```python
from build123d import *

# Parameters (mm, degrees)
SKETCH1_R               = 12.5
SKETCH1_R_2             = 6
BOSS_EXTRUDE1_DEPTH     = 18
SKETCH2_W               = 15
SKETCH2_H               = 15
BOSS_EXTRUDE2_DEPTH     = 25
BOSS_EXTRUDE3_DEPTH     = 20
CHAMFER1_SIZE           = 3
SKETCH4_R               = 5
BOSS_EXTRUDE4_DEPTH     = 15
CUT_EXTRUDE2_DEPTH      = 64.876834612
CUT_EXTRUDE2_DEPTH_BACK = 64.876834612
SKETCH1_3_R             = 6


with BuildPart() as part:
    # Sketch1 → Boss-Extrude1 (new body)
    with BuildSketch(Plane(origin=(0, 0, 0), x_dir=(0, 0, -1), z_dir=(1, 0, 0))):
        Circle(SKETCH1_R)
        Circle(SKETCH1_R_2, mode=Mode.SUBTRACT)
    extrude(amount=BOSS_EXTRUDE1_DEPTH)

    # Sketch2 → Boss-Extrude2 (add)
    with BuildSketch(Plane.XY):
        with Locations((9.060136008, 0)):
            Rectangle(SKETCH2_W, SKETCH2_H)
    extrude(amount=BOSS_EXTRUDE2_DEPTH)

    # Sketch3 → Boss-Extrude3 (add)
    with BuildSketch(Plane.XY.offset(25)):
        Polygon((12.266098975, 5.700421756), (5.666853814, 5.671037358), (2.392678869, -0.058768796), (5.717749085, -5.759190552), (12.316994245, -5.729806154), (15.591169191, 0), align=None)
    extrude(amount=BOSS_EXTRUDE3_DEPTH)

    # Chamfer1
    chamfer1_edges = [part.edges().sort_by_distance(p)[0] for p in [
        (1.560136008, -7.5, 17.5),
        (16.560136008, 7.5, 17.5),
        (1.560136008, 7.5, 17.5),
        (16.560136008, -7.5, 17.5),
    ]]
    chamfer(chamfer1_edges, length=CHAMFER1_SIZE)

    # Sketch4 → Boss-Extrude4 (add)
    with BuildSketch(Plane.XY.offset(45)):
        with Locations((9.066652134, 0)):
            Circle(SKETCH4_R)
    extrude(amount=BOSS_EXTRUDE4_DEPTH)

    # Sketch1<3> → Cut-Extrude2 (cut, two sides: drawn at the far end of the back side and taken through both)
    with BuildSketch(Plane(origin=(0, 0, 0), x_dir=(0, 0, -1), z_dir=(1, 0, 0)).offset(-CUT_EXTRUDE2_DEPTH_BACK)):
        Circle(SKETCH1_3_R)
    extrude(amount=CUT_EXTRUDE2_DEPTH + CUT_EXTRUDE2_DEPTH_BACK, mode=Mode.SUBTRACT)


solid = part.part
```
Here's how the part is built. I have some questions about the finished solid (model axes, mm). A direction names the side the tool comes from. Give positions to 0.01 mm unless a question says otherwise; leave off trailing zeros. Order: outer loops, then holes, each group sorted by start corner. A loop starts at its lowest first (then second) coordinate and runs counter-clockwise, first axis right, second up. Notation, with made-up numbers: (39.5, 66) - (89.5, 66) arc R26 cw to (89.5, 82) - close; hole circle Ø3 at (47, -18.5). An arc over 180 degrees is marked (long way). Answer as a JSON object with one key per item and string values. Group by question number.
Item 1: If we section it at C-C on z = 19.5: Please give me the cut outline in (x, y), and give its area (3 significant figures).
Item 2: If we mould it in two halves opening along Z, with no side actions, what happens to faces 1 (the cylindrical face through (9, 0, 6)), 2 (the flat face through (1.56, 0, 18)), 3 (the flat face through (7, -5, 45))? For each: pulls with the +Z half, pulls with the -Z half, needs draft (parallel to the pull), parting line crosses it, or undercut.
Item 3: For P1, Ø8, axis at y = -1, z = 28, coming from the +X side; P2, Ø3, axis at y = -8.5, z = 37.5, coming from the -X side; P3, Ø7, axis at y = -0.5, z = 17.5, coming from the -X side; P4, Ø4.5, axis at x = 10.5, z = 18.5, coming from the +Y side, each with a flat end and sliding along its axis, tell me the tip position at first contact or that it passes through.
Item 4: Which directions (+Z, -Z, +X, -X, +Y, -Y) give clear straight access to the entire face, cutting with the end or side of a thin tool? Please do faces 4 (the cylindrical face through (7.98, -4.88, 52.4)), 5 (the flat face through (9, 7.5, 17)), 6 (the flat face through (9, -7.5, 17)), 7 (the flat face through (4.053, 2.846, 34.86)), 8 (the flat face through (4.032, -2.869, 34.86)).
Item 5: If we section it at A-A on z = 0: Please give me the cut outline in (x, y).
Item 6: If we section it at D-D on x = 9: Please give me the cut outline in (y, z), and give its area (3 significant figures).
Item 7: Please list where these lines run through material, in increasing order: probe 1 along Y at (x, z) = (4.5, 0); probe 2 along Y at (x, z) = (10.5, -4); probe 3 along Z at (x, y) = (14.75, 1.75).
Item 8: If we section it at B-B on y = 1.5: Please give me the cut outline in (x, z).
Result set:
{
 "1": {"outline": "(1.56, -4.5) - (4.56, -7.5) - (13.56, -7.5) - (16.56, -4.5) - (16.56, 4.5) - (13.56, 7.5) - (4.56, 7.5) - (1.56, 4.5) - close", "area": "207 mm²"},
 "2": {"face 1": "undercut", "face 2": "needs draft", "face 3": "pulls with the +Z half"},
 "3": {"P1": "x = 16.56", "P2": "through", "P3": "x = 1.56", "P4": "y = 7.5"},
 "4": {"face 4": "+Z", "face 5": "+Z, +X, -X, +Y", "face 6": "+Z, +X, -X, -Y", "face 7": "+Z, -X, +Y", "face 8": "+Z, -X, -Y"},
 "5": {"outline": "(0, -12.5) - (18, -12.5) - (18, -6) - (0, -6) - close; (0, 6) - (18, 6) - (18, 12.5) - (0, 12.5) - close"},
 "6": {"outline": "(-7.5, 10) arc R12.5 ccw (long way) to (7.5, 10) - (7.5, 25) - (5.69, 25) - (5.69, 45) - (5, 45) - (5, 60) - (-5, 60) - (-5, 45) - (-5.74, 45) - (-5.74, 25) - (-7.5, 25) - close; hole circle Ø12 at (0, 0)", "area": "956 mm²"},
 "7": {"probe 1": "-12.5 to -6, 6 to 12.5", "probe 2": "-11.84 to -4.47, 4.47 to 11.84", "probe 3": "-12.38 to -5.74, 5.74 to 25"},
 "8": {"outline": "(0, -12.41) - (18, -12.41) - (18, -5.81) - (0, -5.81) - close; (0, 5.81) - (18, 5.81) - (18, 12.41) - (16.56, 12.41) - (16.56, 25) - (14.72, 25) - (14.72, 45) - (13.84, 45) - (13.84, 60) - (4.3, 60) - (4.3, 45) - (3.28, 45) - (3.28, 25) - (1.56, 25) - (1.56, 12.41) - (0, 12.41) - close"}
}
